```python
from build123d import *

# Parameters (mm, degrees)
SKETCH1_R           = 1.6
BOSS_EXTRUDE1_DEPTH = 5
SKETCH2_R           = 1.6
BOSS_EXTRUDE2_DEPTH = 5
SKETCH3_R           = 1.6
BOSS_EXTRUDE3_DEPTH = 5


with BuildPart() as part:
    # Sketch1 → Boss-Extrude1 (new body)
    with BuildSketch(Plane(origin=(0, 0, 0), x_dir=(1, 0, 0), z_dir=(0, 1, 0))):
        with BuildLine():
            Line((-50, 0), (-60, 0))
            Line((-60, 0), (-60, 15))
            Line((-60, 15), (15, 15))
            Line((15, 15), (15, -60))
            Line((15, -60), (0, -60))
            Line((0, -60), (0, -50))
            ThreePointArc((0, -50), (-14.644660941, -14.644660941), (-50, 0))
        make_face()
        with Locations(Location((7.5, 7.5, 0), (0, 0, 270))):
            Circle(SKETCH1_R, mode=Mode.SUBTRACT)
        with Locations(Location((7.5, -6.6, 0), (0, 0, 270))):
            Circle(SKETCH1_R, mode=Mode.SUBTRACT)
        with Locations(Location((7.5, -53.4, 0), (0, 0, 270))):
            Circle(SKETCH1_R, mode=Mode.SUBTRACT)
        with Locations(Location((-53.4, 7.5, 0), (0, 0, 270))):
            Circle(SKETCH1_R, mode=Mode.SUBTRACT)
        with Locations(Location((-6.6, 7.5, 0), (0, 0, 270))):
            Circle(SKETCH1_R, mode=Mode.SUBTRACT)
    extrude(amount=BOSS_EXTRUDE1_DEPTH)

    # Sketch2 → Boss-Extrude2 (add)
    with BuildSketch(Plane(origin=(15, 0, 0), x_dir=(0, 0, -1), z_dir=(1, 0, 0))):
        with BuildLine():
            Line((-10, -10), (-20, 0))
            Line((-20, 0), (-60, 0))
            Line((-60, 0), (-60, 15))
            ThreePointArc((-60, 15), (-58.535533906, 18.535533906), (-55, 20))
            Line((-55, 20), (-45, 20))
            ThreePointArc((-45, 20), (-13.180194847, 33.180194847), (0, 65))
            Line((0, 65), (0, 70))
            ThreePointArc((0, 70), (1.464466094, 73.535533906), (5, 75))
            Line((5, 75), (15, 75))
            Line((15, 75), (15, -10))
            Line((15, -10), (-10, -10))
        make_face()
        with Locations((-53.4, 12.5)):
            Circle(SKETCH2_R, mode=Mode.SUBTRACT)
        with Locations((-6.6, 12.5)):
            Circle(SKETCH2_R, mode=Mode.SUBTRACT)
        with Locations((7.5, 26.6)):
            Circle(SKETCH2_R, mode=Mode.SUBTRACT)
        with Locations((7.5, 68.4)):
            Circle(SKETCH2_R, mode=Mode.SUBTRACT)
    extrude(amount=BOSS_EXTRUDE2_DEPTH)

    # Sketch3 → Boss-Extrude3 (add)
    with BuildSketch(Plane(origin=(0, 0, -15), x_dir=(-1, 0, 0), z_dir=(0, 0, -1))):
        with BuildLine():
            Line((-20, -10), (10, -10))
            Line((10, -10), (20, 0))
            Line((20, 0), (60, 0))
            Line((60, 0), (60, 15))
            ThreePointArc((60, 15), (58.535533906, 18.535533906), (55, 20))
            Line((55, 20), (45, 20))
            ThreePointArc((45, 20), (13.180194847, 33.180194847), (0, 65))
            Line((0, 65), (0, 70))
            ThreePointArc((0, 70), (-1.464466094, 73.535533906), (-5, 75))
            Line((-5, 75), (-20, 75))
            Line((-20, 75), (-20, -10))
        make_face()
        with Locations((-7.5, 68.4)):
            Circle(SKETCH3_R, mode=Mode.SUBTRACT)
        with Locations((-7.5, 26.6)):
            Circle(SKETCH3_R, mode=Mode.SUBTRACT)
        with Locations((6.6, 12.5)):
            Circle(SKETCH3_R, mode=Mode.SUBTRACT)
        with Locations((53.4, 12.5)):
            Circle(SKETCH3_R, mode=Mode.SUBTRACT)
    extrude(amount=BOSS_EXTRUDE3_DEPTH)


solid = part.part
```
Check sheet for the modelled part. Datum: model origin and axes. Units: mm. A direction names the side the tool comes from. Round coordinates to 2 decimals unless told otherwise and drop trailing zeros. Order: outer loops, then holes, each group sorted by start corner. A loop starts at its lowest first (then second) coordinate and runs counter-clockwise, first axis right, second up.
1) Section check B-B (x = 7.5). Record the boundary of the cut face in (y, z).
2) Section check A-A (y = 68.4). Record the boundary of the cut face in (x, z).
3) Mould release check, pull along X, two halves, no side actions. Record for faces 1 (the cylindrical face through (5.94, 2.46, -7.85)), 2 (the flat face through (-2, 24, -20)), 3 (the cylindrical face through (-14.258, 2.465, 15.036)): +X half, -X half, draft (parallel to the pull), parting line (faces both ways), or undercut.
4) Tool access check on faces 4 (the flat face through (0, 2, 55)), 5 (the flat face through (0, 67, -17)), 6 (the flat face through (17, 20, 50)), 7 (the flat face through (2, -5, -15)). Record the directions out of +Z, -Z, +X, -X, +Y, -Y that give a thin tool (end or side, any length) a straight path to the whole face; none if there is none.
5) Go/stop test with flat-tipped pins: pin 1 Ø5 at (x, z) = (7.5, 6.6) entering from +Y; pin 2 Ø5 at (y, z) = (-4, 1) entering from -X; pin 3 Ø1.9 at (x, z) = (7.5, 53.4) entering from +Y; pin 4 Ø4 at (x, y) = (7.5, 68.4) entering from -Z. Record where each tip stops, or that it passes through.
6) Section check D-D (y = 12.5). Record the boundary of the cut face in (x, z), and give its area (3 significant figures).
7) Scan lines: line 1 (X direction, y = 3, z = -7.5); line 2 (Z direction, x = 7, y = 3); line 3 (Y direction, x = 0.5, z = 12). Record each from-to range of solid material in increasing order.
8) Section check C-C (z = -7.5). Record the boundary of the cut face in (x, y).
Result:
1. outline: (-10, -20) - (25, -20) - (25, -15) - (5, -15) - (5, -9.1) - (0, -9.1) - (0, -15) - (-10, -15) - close; (0, -5.9) - (5, -5.9) - (5, 5) - (0, 5) - close; (0, 8.2) - (5, 8.2) - (5, 51.8) - (0, 51.8) - close; (0, 55) - (5, 55) - (5, 60) - (0, 60) - close; (28.2, -20) - (66.8, -20) - (66.8, -15) - (28.2, -15) - close; (70, -20) - (75, -20) - (75, -15) - (70, -15) - close
2. outline: (0, -20) - (5.9, -20) - (5.9, -15) - (0, -15) - close; (9.1, -20) - (20, -20) - (20, -9.1) - (15, -9.1) - (15, -15) - (9.1, -15) - close; (15, -5.9) - (20, -5.9) - (20, 0) - (15, 0) - close
3. face 1: undercut
3. face 2: draft
3. face 3: -X half
4. face 4: +Z, -X, +Y, -Y
4. face 5: +Z, -Z, -X, +Y
4. face 6: +Z, +X, -X, +Y
4. face 7: +Z, -X, -Y
5. pin 1: stops at y = 5
5. pin 2: stops at x = 15
5. pin 3: passes through
5. pin 4: stops at z = -20
6. outline: (-60, -20) - (-55, -20) - (-55, -15) - (-60, -15) - close; (-51.8, -20) - (-8.2, -20) - (-8.2, -15) - (-51.8, -15) - close; (-5, -20) - (20, -20) - (20, 5) - (15, 5) - (15, -15) - (-5, -15) - close; (15, 8.2) - (20, 8.2) - (20, 51.8) - (15, 51.8) - close; (15, 55) - (20, 55) - (20, 60) - (15, 60) - close
6. area: 711 mm2
7. line 1: x = -60 to -55, -51.8 to -8.2, -5 to 5.9, 9.1 to 20
7. line 2: z = -20 to -9.02, -5.98 to 5.08, 8.12 to 51.88, 54.92 to 60
7. line 3: y = 0 to 5
8. outline: (-60, 0) - (-55, 0) - (-55, 5) - (-60, 5) - close; (-51.8, 0) - (-8.2, 0) - (-8.2, 5) - (-51.8, 5) - close; (-5, 0) - (5.9, 0) - (5.9, 5) - (-5, 5) - close; (9.1, 0) - (15, 0) - (15, -10) - (20, -10) - (20, 25) - (15, 25) - (15, 5) - (9.1, 5) - close; (15, 28.2) - (20, 28.2) - (20, 66.8) - (15, 66.8) - close; (15, 70) - (20, 70) - (20, 75) - (15, 75) - close
